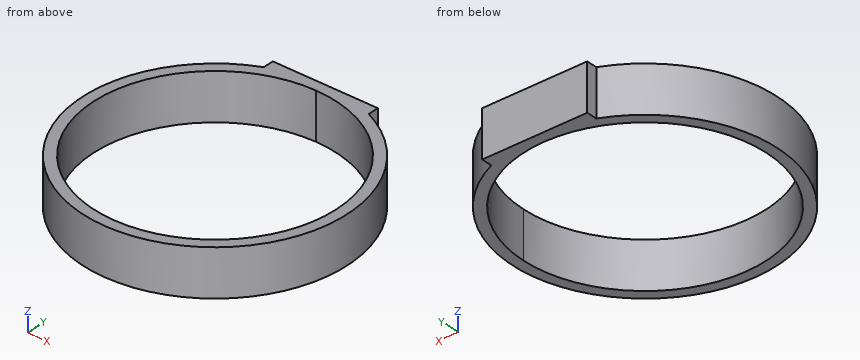
from build123d import *

# Parameters (mm, degrees)
IZIM1_R                     = 85
IZIM1_R_2                   = 78
Y_KSEKLIK_EKSTR_ZYON1_DEPTH = 15
IZIM2_W                     = 67.56
IZIM2_H                     = 7.000566669
Y_KSEKLIK_EKSTR_ZYON2_DEPTH = 30


with BuildPart() as part:
    # Çizim1 → Yükseklik-Ekstrüzyon1 (new, symmetric)
    with BuildSketch(Plane.XY):
        Circle(IZIM1_R)
        Circle(IZIM1_R_2, mode=Mode.SUBTRACT)
    extrude(amount=Y_KSEKLIK_EKSTR_ZYON1_DEPTH, both=True)

    # Çizim2 → Yükseklik-Ekstrüzyon2 (add)
    with BuildSketch(Plane.XY.offset(15)):
        with Locations((0, 81.499716666)):
            Rectangle(IZIM2_W, IZIM2_H)
    extrude(amount=-Y_KSEKLIK_EKSTR_ZYON2_DEPTH)


solid = part.part
Can you work these out from the model? Positions are in its coordinate system, mm. Give positions to 0.01 mm unless a question says otherwise; leave off trailing zeros. Loops run counter-clockwise (first coordinate to the right, second up) from the corner with the lowest first, then second, coordinate; pieces in that order, holes last. Notation, with made-up numbers: (51.25, 56.5) -> (105.25, 56.5) arc R25 cw to (105.25, 69.5) -> close; hole circle Ø2 at (28.25, 62.5). An arc over 180 degrees is marked (long way). Return JSON: item names as keys, results as strings.
Q1. I want a section at A-A, the plane z = -11.5. List the corners of the cut face in (x, y) for me, then the cut area to 3 significant figures.
Checks:
{"outline": "(-33.78, 78) arc R85 ccw (long way) to (33.78, 78) -> (33.78, 85) -> (-33.78, 85) -> close; hole (-0.3, 78) arc R78 ccw (long way) to (0.3, 78) -> close", "area": "3,740 mm2"}
Q2. I want a section at B-B, the plane y = -21.5. List the corners of the cut face in (x, z) for me, then the cut area to 3 significant figures.
Checks:
{"outline": "(-82.24, -15) -> (-74.98, -15) -> (-74.98, 15) -> (-82.24, 15) -> close; (74.98, -15) -> (82.24, -15) -> (82.24, 15) -> (74.98, 15) -> close", "area": "435 mm2"}
Q3. I want a section at C-C, the plane x = 51. List the corners of the cut face in (y, z) for me.
Checks:
{"outline": "(-68, -15) -> (-59.02, -15) -> (-59.02, 15) -> (-68, 15) -> close; (59.02, -15) -> (68, -15) -> (68, 15) -> (59.02, 15) -> close"}
Q4. For pin 1 Ø3 at (x, z) = (-54.5, -10) entering from +Y; pin 2 Ø2 at (y, z) = (82.5, 1) entering from -X; pin 3 Ø3 at (x, z) = (57, 6) entering from +Y, each with a flat end and sliding along its axis, tell me the tip position at first contact or that it passes through.
Checks:
{"pin 1": "stops at y = 66.45", "pin 2": "stops at x = -33.78", "pin 3": "stops at y = 64.38"}
Q5. I need wall thicknesses on probe 1 along X at (y, z) = (0, -3); probe 2 along X at (y, z) = (37, 13.75). Which ranges of each line are inside material? Lowest first, please.
Checks:
{"probe 1": "x = -85 to -78, 78 to 85", "probe 2": "x = -76.52 to -68.67, 68.67 to 76.52"}
